Autodesk Inventor part; units mm, degrees
ref_plane "YZ Plane" through (0, 0, 0) normal (1, 0, 0) x (0, 1, 0)
ref_plane "XZ Plane" through (0, 0, 0) normal (0, 1, 0) x (-1, 0, 0)
ref_plane "XY Plane" through (0, 0, 0) normal (0, 0, 1) x (1, 0, 0)
sketch "Sketch1" plane through (0, 0, 0) normal (0, 1, 0) x (-1, 0, 0)
  circle A0 centre (25.8401, 17.3142) radius 1.75
  point P0 (0, 0)
  dimension "d0" = 3.5
extrude "Extrusion1" add sketch "Sketch1" along normal blind 4
thread "Thread1"
sketch "Sketch2" plane through (-25.8401, 4, 17.3142) normal (0, 1, 0) x (1, 0, 0)
  circle A0 centre (0, 0) radius 2.5
  point P0 (25.8401, 17.3142)
  dimension "d5" = 5
extrude "Extrusion2" add sketch "Sketch2" along normal blind 1.5
fillet "Fillet1" radius 2 1 edges at (-28.3401, 5.5, 17.3142)
properties part number "screwLarge"
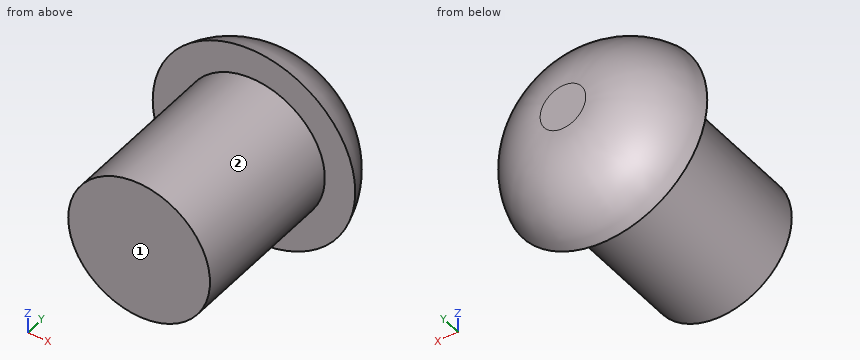
Input: part model. Units: mm. Frame: model coordinates. Face numbers are marked on the shaded views. A direction names the side the tool comes from. Give positions to 0.01 mm unless a question says otherwise; leave off trailing zeros. Order: outer loops, then holes, each group sorted by start corner. A loop starts at its lowest first (then second) coordinate and runs counter-clockwise, first axis right, second up. Notation, with made-up numbers: (19.25, -38) - (41.25, -38) arc R31 ccw to (41.25, -10) - close; hole circle Ø11 at (7, 48.25). An arc over 180 degrees is marked (long way). Use a Markdown table: item, result.
(1) Section query A-A (y = 3.85). Output: boundary loops of the cut face in (x, z), then the cut area to 3 significant figures.
Computed values:
| item | result |
|---|---|
| outline | circle Ø3.5 at (-25.84, 17.31) |
| area | 9.62 mm2 |
(2) Pin query (flat end, axial travel): pin 1 (1 mm diameter, centred on x = -27, z = 16.5, fed in from +Y). Return the tip coordinate at first contact, or that it passes through.
Computed values:
| item | result |
|---|---|
| pin 1 | stops at y = 5.47 |
(3) Access query for the marked faces 1 and 2. Directions: +Z, -Z, +X, -X, +Y, -Y. A direction counts if a zero-diameter tool reaches every point of the face in a straight line with its end or side. Return the directions, or none.
Computed values:
| item | result |
|---|---|
| face 1 | +Z, -Z, +X, -X, -Y |
| face 2 | -Y |
(4) Line query: line 1 (X direction, y = 3.95, z = 18.3); line 2 (Y direction, x = -27.85, z = 16.75); line 3 (X direction, y = 4.75, z = 19.1). Output: solid intervals per line, ascending. Write a range as from..to.
Computed values:
| item | result |
|---|---|
| line 1 | x = -27.29..-24.39 |
| line 2 | y = 4..4.8 |
| line 3 | x = -26.99..-24.69 |
